For this review, take the finished solid that the model builds, in its own axes (mm). A direction names the side the tool comes from. Round coordinates to 2 decimals unless told otherwise and drop trailing zeros. Write each loop counter-clockwise with the first axis right and the second up, starting at its lowest first coordinate (ties: lowest second). Pieces come first, ordered by that corner, then holes.
from build123d import *

# Parameters (mm, degrees)
F0_W     = 40
F0_H     = 6
F1_DEPTH = 37
F2_DEPTH = 5
F3_DEPTH = 31
F4_DEPTH = 25
F5_DEPTH = 20


with BuildPart() as f1:
    # F0 (on Front) → F1 (new body)
    with BuildSketch(Plane.XZ):
        with Locations((-14.9053405225, 48.0189405978)):
            Rectangle(F0_W, F0_H)
    extrude(amount=F1_DEPTH)

    # F0 (on Front) → F2 (join)
    with BuildSketch(Plane.XZ):
        with BuildLine():
            Line((5.0946594775, -37.9810594022), (5.0946594775, 45.0189405978))
            Line((5.0946594775, 45.0189405978), (-34.9053405225, 45.0189405978))
            Line((-34.9053405225, 45.0189405978), (-34.9053405225, -37.9810594022))
            Line((-34.9053405225, -37.9810594022), (-27.4053405225, -37.9810594022))
            ThreePointArc((-27.4053405225, -37.9810594022), (-14.9053405225, -25.4810594022), (-2.4053405225, -37.9810594022))
            Line((-2.4053405225, -37.9810594022), (5.0946594775, -37.9810594022))
        make_face()
        with BuildLine():
            ThreePointArc((-34.9053405225, -37.9810594022), (-14.9053405225, -57.9810594022), (5.0946594775, -37.9810594022))
            Line((5.0946594775, -37.9810594022), (-2.4053405225, -37.9810594022))
            ThreePointArc((-2.4053405225, -37.9810594022), (-14.9053405225, -50.4810594022), (-27.4053405225, -37.9810594022))
            Line((-27.4053405225, -37.9810594022), (-34.9053405225, -37.9810594022))
        make_face()
    extrude(amount=F2_DEPTH)

    # F0 (on Front) → F3 (join)
    with BuildSketch(Plane.XZ):
        with BuildLine():
            Line((5.0946594775, 76.0189405978), (-6.9053405225, 76.0189405978))
            ThreePointArc((-6.9053405225, 76.0189405978), (-14.9053405225, 68.0189405978), (-22.9053405225, 76.0189405978))
            Line((-22.9053405225, 76.0189405978), (-34.9053405225, 76.0189405978))
            Line((-34.9053405225, 76.0189405978), (-34.9053405225, 51.0189405978))
            Line((-34.9053405225, 51.0189405978), (5.0946594775, 51.0189405978))
            Line((5.0946594775, 51.0189405978), (5.0946594775, 76.0189405978))
        make_face()
        with BuildLine():
            ThreePointArc((-22.9053405225, 76.0189405978), (-14.9053405225, 84.0189405978), (-6.9053405225, 76.0189405978))
            Line((-6.9053405225, 76.0189405978), (5.0946594775, 76.0189405978))
            ThreePointArc((5.0946594775, 76.0189405978), (-14.9053405225, 96.0189405978), (-34.9053405225, 76.0189405978))
            Line((-34.9053405225, 76.0189405978), (-22.9053405225, 76.0189405978))
        make_face()
    extrude(amount=F3_DEPTH)

    # F0 (on Front) → F4 (cut)
    with BuildSketch(Plane.XZ):
        with BuildLine():
            Line((5.0946594775, 76.0189405978), (-6.9053405225, 76.0189405978))
            ThreePointArc((-6.9053405225, 76.0189405978), (-14.9053405225, 68.0189405978), (-22.9053405225, 76.0189405978))
            Line((-22.9053405225, 76.0189405978), (-34.9053405225, 76.0189405978))
            Line((-34.9053405225, 76.0189405978), (-34.9053405225, 51.0189405978))
            Line((-34.9053405225, 51.0189405978), (5.0946594775, 51.0189405978))
            Line((5.0946594775, 51.0189405978), (5.0946594775, 76.0189405978))
        make_face()
        with BuildLine():
            ThreePointArc((-22.9053405225, 76.0189405978), (-14.9053405225, 84.0189405978), (-6.9053405225, 76.0189405978))
            Line((-6.9053405225, 76.0189405978), (5.0946594775, 76.0189405978))
            ThreePointArc((5.0946594775, 76.0189405978), (-14.9053405225, 96.0189405978), (-34.9053405225, 76.0189405978))
            Line((-34.9053405225, 76.0189405978), (-22.9053405225, 76.0189405978))
        make_face()
    extrude(amount=F4_DEPTH, mode=Mode.SUBTRACT)

    # F0 (on Front) → F5 (join)
    with BuildSketch(Plane.XZ):
        with BuildLine():
            Line((-6.9053405225, -37.9810594022), (-2.4053405225, -37.9810594022))
            ThreePointArc((-2.4053405225, -37.9810594022), (-14.9053405225, -25.4810594022), (-27.4053405225, -37.9810594022))
            Line((-27.4053405225, -37.9810594022), (-22.9053405225, -37.9810594022))
            ThreePointArc((-22.9053405225, -37.9810594022), (-14.9053405225, -29.9810594022), (-6.9053405225, -37.9810594022))
        make_face()
        with BuildLine():
            ThreePointArc((-27.4053405225, -37.9810594022), (-14.9053405225, -50.4810594022), (-2.4053405225, -37.9810594022))
            Line((-2.4053405225, -37.9810594022), (-6.9053405225, -37.9810594022))
            ThreePointArc((-6.9053405225, -37.9810594022), (-14.9053405225, -45.9810594022), (-22.9053405225, -37.9810594022))
            Line((-22.9053405225, -37.9810594022), (-27.4053405225, -37.9810594022))
        make_face()
    extrude(amount=F5_DEPTH)

    # F6: F1 across plane


with BuildPart() as f1_1:
    add(f1.part)
    add(f1.part.mirror(Plane.XZ))


solid = f1_1.part
(1) For line 1 along Z through (x, y) = (-14.5, -8.5); line 2 along Y through (x, z) = (-32, 68); line 3 along Z through (x, y) = (-11, 10.5), list the stretches that pass through material, from the lowest coordinate up.
Geometry check:
line 1: z = -50.47 to -45.97, -29.99 to -25.49, 45.02 to 51.02
line 2: y = -31 to -25, 25 to 31
line 3: z = -49.86 to -44.96, -31 to -26.11, 45.02 to 51.02
(2) We need section A-A, the plane y = -14. Give the boundary of the cut face in (x, z).
Geometry check:
outline: (-34.91, 45.02) - (5.09, 45.02) - (5.09, 51.02) - (-34.91, 51.02) - close; circle Ø25 at (-14.91, -37.98); hole circle Ø16 at (-14.91, -37.98)
(3) For faces 4 (the face through (-15, 21, 45.019)), 5 (the face through (-15, 34, 51.019)), 6 (the face through (-10.7, 25, 68.8)), list the 3-axis set-ups (+Z, -Z, +X, -X, +Y, -Y) from which the entire face can be reached by the end or side of a thin tool; tool diameter is ignored.
Geometry check:
face 4: +X, -X, +Y
face 5: +Z, +X, -X, +Y
face 6: +Z, +X, -X
(4) For pin 1 Ø6.5 at (x, y) = (-22, -34.5) entering from +Z; pin 2 Ø12 at (x, y) = (-12, -29) entering from -Z; pin 3 Ø20 at (x, z) = (-13.5, 0) entering from +Y; pin 4 Ø12 at (y, z) = (7, -41) entering from +X, all flat-tipped, find the tip position at first contact; note any pin that passes through.
Geometry check:
pin 1: stops at z = 51.02
pin 2: stops at z = 45.02
pin 3: stops at y = 5
pin 4: stops at x = 5.09
(5) We need section D-D, the plane y = -22. Give the boundary of the cut face in (x, z), and give its area (3 significant figures).
Geometry check:
outline: (-34.91, 45.02) - (5.09, 45.02) - (5.09, 51.02) - (-34.91, 51.02) - close
area: 240 mm2
(6) We need section B-B, the plane z = 71. Give the boundary of the cut face in (x, y), and give its area (3 significant figures).
Geometry check:
outline: (-34.91, -31) - (-21.14, -31) - (-21.14, -25) - (-34.91, -25) - close; (-34.91, 25) - (-21.14, 25) - (-21.14, 31) - (-34.91, 31) - close; (-8.68, -31) - (5.09, -31) - (5.09, -25) - (-8.68, -25) - close; (-8.68, 25) - (5.09, 25) - (5.09, 31) - (-8.68, 31) - close
area: 330 mm2
(7) Mouldability with a two-part tool opening along X and no side actions: class faces 1 (the face through (-34.905, 0, 28)), 2 (the face through (-13.86, 27.96, 83.95)), 3 (the face through (-15, -21, 45.019)) as pulls with the +X half, pulls with the -X half, needs draft (parallel to the pull), parting line crosses it, or undercut.
Geometry check:
face 1: pulls with the -X half
face 2: undercut
face 3: needs draft
(8) We need section C-C, the plane x = -26. Give the boundary of the cut face in (y, z), and give its area (3 significant figures).
Geometry check:
outline: (-37, 45.02) - (-5, 45.02) - (-5, -32.22) - (-20, -32.22) - (-20, -43.74) - (-5, -43.74) - (-5, -54.62) - (5, -54.62) - (5, -43.74) - (20, -43.74) - (20, -32.22) - (5, -32.22) - (5, 45.02) - (37, 45.02) - (37, 51.02) - (31, 51.02) - (31, 92.66) - (25, 92.66) - (25, 51.02) - (-25, 51.02) - (-25, 92.66) - (-31, 92.66) - (-31, 51.02) - (-37, 51.02) - close
area: 2,290 mm2
